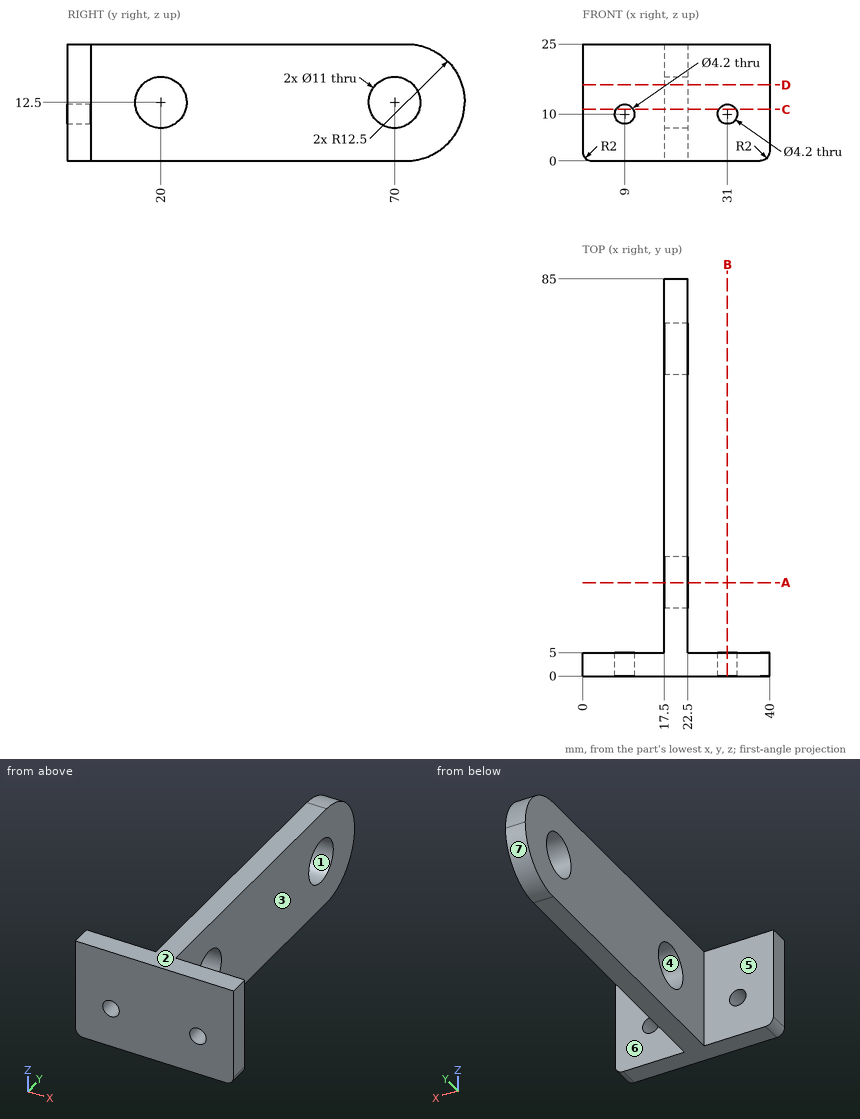
The figure shows three views and two pictorial views of one solid part (mm, origin at its lowest corner). Answer the questions. A direction names the side the tool comes from. Give positions to 0.01 mm unless a question says otherwise; leave off trailing zeros. Write each loop counter-clockwise with the first axis right and the second up, starting at its lowest first coordinate (ties: lowest second). Pieces come first, ordered by that corner, then holes. Notation, with made-up numbers: (-23, -24.75) - (10, -24.75) arc R15 cw to (10, -17.75) - close; hole circle Ø5 at (-5.5, 69). An arc over 180 degrees is marked (long way). Use one line per item in the form item = value.
1. Consider L1, parallel to X at y = 2.1, z = 10; L2, parallel to Y at x = 19.8, z = 12.5; L3, parallel to Y at x = 3.5, z = 9. Determine where each line is inside the solid, lowest interval first.
Filled in:
L1 = 0 to 6.9, 11.1 to 28.9, 33.1 to 40
L2 = 0 to 14.5, 25.5 to 64.5, 75.5 to 85
L3 = 0 to 5
2. A cutting plane is placed at B-B (x = 31). Write down the section's boundary in (y, z), and give its area (3 significant figures).
Filled in:
outline = (0, 0) - (5, 0) - (5, 7.9) - (0, 7.9) - close; (0, 12.1) - (5, 12.1) - (5, 25) - (0, 25) - close
area = 104 mm^2
3. A cutting plane is placed at D-D (z = 16.25). Write down the section's boundary in (x, y).
Filled in:
outline = (0, 0) - (40, 0) - (40, 5) - (22.5, 5) - (22.5, 15.98) - (17.5, 15.98) - (17.5, 5) - (0, 5) - close; (17.5, 24.02) - (22.5, 24.02) - (22.5, 65.98) - (17.5, 65.98) - close; (17.5, 74.02) - (22.5, 74.02) - (22.5, 84.42) - (17.5, 84.42) - close
4. For the marked faces 5, 6 and 7, determine the directions among +Z, -Z, +X, -X, +Y, -Y from which every point of the face is accessible in a straight line to the end or side of a thin tool.
Filled in:
face_5 = +Z, -Z, -X, +Y
face_6 = +Z, -Z, +X, +Y
face_7 = -Z, +X, -X, +Y
5. Each of these flat-tipped pins is pushed along its axis until it touches: pin 1 Ø2 at (y, z) = (20.5, 21) entering from +X; pin 2 Ø5 at (x, z) = (30, 17) entering from +Y; pin 3 Ø4 at (y, z) = (56, 3) entering from -X; pin 4 Ø1.5 at (x, y) = (15.5, 36) entering from -Z. Where does it stop, or does it pass through?
Filled in:
pin_1 = 22.5
pin_2 = 5
pin_3 = 17.5
pin_4 = through
6. A cutting plane is placed at C-C (z = 11). Write down the section's boundary in (x, y), and give its area (3 significant figures).
Filled in:
outline = (0, 0) - (7.15, 0) - (7.15, 5) - (0, 5) - close; (10.85, 0) - (29.15, 0) - (29.15, 5) - (22.5, 5) - (22.5, 14.71) - (17.5, 14.71) - (17.5, 5) - (10.85, 5) - close; (17.5, 25.29) - (22.5, 25.29) - (22.5, 64.71) - (17.5, 64.71) - close; (17.5, 75.29) - (22.5, 75.29) - (22.5, 84.91) - (17.5, 84.91) - close; (32.85, 0) - (40, 0) - (40, 5) - (32.85, 5) - close
area = 457 mm^2
7. Determine the mould class of the marked faces 1, 2, 3 and 4 for opening direction Z: released by +Z, released by -Z, zero draft, split by the parting line, or undercut.
Filled in:
face_1 = undercut
face_2 = released by +Z
face_3 = zero draft
face_4 = undercut
8. A cutting plane is placed at A-A (y = 20). Write down the section's boundary in (x, z), and give its area (3 significant figures).
Filled in:
outline = (17.5, 0) - (22.5, 0) - (22.5, 7) - (17.5, 7) - close; (17.5, 18) - (22.5, 18) - (22.5, 25) - (17.5, 25) - close
area = 70.0 mm^2
